Input: part model. Units: mm. Frame: model coordinates. A direction names the side the tool comes from. Round coordinates to 2 decimals unless told otherwise and drop trailing zeros. Loops run counter-clockwise (first coordinate to the right, second up) from the corner with the lowest first, then second, coordinate; pieces in that order, holes last. Notation, with made-up numbers: M -19,19.5 L 11,19.5 A11 ccw 11,26.5 Z; hole C 45,77.5 d5. An arc over 180 degrees is marked long. Put each result on its own line as item: value. Start each with the question number.
1) Line query: probe 1 along Y at (x, z) = (0, 18.75); probe 2 along Z at (x, y) = (-26, 22.5); probe 3 along X at (y, z) = (2.5, 0). Output: solid intervals per line, ascending.
2) Section D-D on x = 0. State how many separate pieces and enclosed holes the cut face has, plus the area to 3 significant figures.
3) Section C-C on x = 19. Output: boundary loops of the cut face in (y, z).
4) Section A-A on z = 0. Output: boundary loops of the cut face in (x, y), plus the area to 3 significant figures.
5) Pin query (flat end, axial travel): pin 1 (4 mm diameter, centred on y = 16.5, z = 15, fed in from -X); pin 2 (22 mm diameter, centred on x = 21, z = -1.5, fed in from +Y); pin 3 (16 mm diameter, centred on x = -21, z = 2, fed in from +Y). Return the tip coordinate at first contact, or that it passes through.
6) Draft query along Z for faces 1 (the face through (0, 15, 22.5)), 2 (the face through (22.057, 10.804, 15.789)), 3 (the face through (-8, 0, -15)). Return one class per face: +Z half, -Z half, draft (parallel to the pull), parting line (faces both ways), or undercut.
7) Reachability of faces 4 (the face through (19.2, 27.98, 20.04)), 5 (the face through (-21.775, 10.711, -15.696)) from +Z, -Z, +X, -X, +Y, -Y: full face, straight path, thin tool, end or side. Return the list, or none.
8) Section B-B on y = 22.22. Output: boundary loops of the cut face in (x, z).
Autodesk Fusion 360 part; units mm, degrees
sketch "Sketch1" plane through (0, 0, 0) normal (0, 1, 0) x (1, 0, 0)
  line L0 (32, -22.5) -> (-32, -22.5)
  line L1 (-32, -22.5) -> (-32, 22.5)
  line L2 (-32, 22.5) -> (32, 22.5)
  line L3 (32, 22.5) -> (32, -22.5)
  line L4 (32, -22.5) -> (-32, 22.5) construction
  line L5 (-32, -22.5) -> (32, 22.5) construction
  dimension "d1" = 64
  dimension "d6" = 45
extrude "Extrude1" add sketch "Sketch1" along normal blind 40
sketch "Sketch2" plane through (0, 0, 22.5) normal (0, 0, 1) x (-1, 0, 0)
  line L0 (32, 0) -> (-32, 0)
  line L1 (-32, 0) -> (-32, -40)
  line L2 (-32, -40) -> (32, -40)
  line L3 (32, -40) -> (32, 0)
  circle A0 centre (0, -29) radius 11
  line L4 (32, -16) -> (18.8835, -16)
  line L5 (18.8835, -16) -> (-32, -16)
  line L6 (6.7633, -37.6751) -> (32, -18)
  line L7 (-6.7633, -37.6751) -> (-32, -18)
  line L8 (0, 0) -> (0, -40) construction
  line L9 (32, -18) -> (-32, -18)
  dimension "d4" = 22
  dimension "d5" = 24
  dimension "d7" = 22
extrude "Extrude2" cut sketch "Sketch2" against normal blind 45 contours L2 L3 A0 L6 | L1 L2 A0 L7
sketch "Sketch3" plane through (-32, 0, 0) normal (-1, 0, 0) x (0, -1, 0)
  line L0 (-18, 22.5) -> (-18, -22.5)
  line L1 (-18, -22.5) -> (0, -22.5)
  line L2 (0, -22.5) -> (0, 22.5)
  line L3 (0, 22.5) -> (-18, 22.5)
  line L4 (0, 0) -> (-40.0524, 0)
  line L5 (-40, 22.5) -> (-40, -22.5)
  line L6 (-40, -22.5) -> (-37.6751, -22.5)
  line L7 (-37.6751, 22.5) -> (-40, 22.5)
  line L8 (-40, 17.5) -> (-9, 17.5)
  line L9 (-9, 17.5) -> (-9, -17.5)
  line L10 (-9, -17.5) -> (-40, -17.5)
  line L11 (-40, -17.5) -> (-40, 17.5)
  line L12 (-40, 17.5) -> (-9, -17.5) construction
  line L13 (-9, 17.5) -> (-40, -17.5) construction
  point P0 (-24.5, 0)
  dimension "d10" = 35
  dimension "d11" = 31
extrude "Extrude3" cut sketch "Sketch3" against normal blind 64 contours L0 L4 L8 L9 | L0 L4 L5 L8 L11 | L0 L4 L9 L10 | L0 L4 L5 L10 L11
sketch "Sketch4" plane through (0, 0, 22.5) normal (0, 0, 1) x (-1, 0, 0)
  line L0 (6.7633, -37.6751) -> (32, -18)
  line L1 (32, -18) -> (32, 0)
  line L2 (32, 0) -> (-32, 0)
  line L3 (-32, 0) -> (-32, -18)
  line L4 (-32, -18) -> (-6.7633, -37.6751)
  arc A0 (-6.7633, -37.6751) -> (6.7633, -37.6751) centre (0, -29) ccw
  circle A1 centre (0, -29) radius 11
  circle A2 centre (0, -29) radius 3.175
  line L5 (0, -40) -> (0, 0)
  point P0 (0, -34.92)
  point P1 (0, -22.22)
  dimension "d14" = 22
  dimension "d15" = 6.35
  dimension "d18" = 12.7
  dimension "d19" = 5.08
hole "Hole1" at (0, 22.22, 22.5) at (0, 34.92, 22.5) direction (0, 0, -1) diameter 6.5 depth 49 tip angle 180
sketch "Sketch5" plane through (0, 0, 0) normal (0, -1, 0) x (1, 0, 0)
  line L0 (-32, -22.5) -> (32, -22.5)
  line L1 (32, -22.5) -> (32, 22.5)
  line L2 (32, 22.5) -> (-32, 22.5)
  line L3 (-32, 22.5) -> (-32, -22.5)
  circle A0 centre (0, 0) radius 16.5
  dimension "d23" = 33
extrude "Extrude5" cut sketch "Sketch5" against normal blind 9 contours A0
fillet "Fillet1" radius 6 2 edges at (0, 9, -17.5) (0, 9, 17.5)
Geometry results:
1. probe 1: y = 0 to 18.97, 25.47 to 31.67, 38.17 to 40
1. probe 2: z = -22.5 to -17.5, 17.5 to 22.5
1. probe 3: x = -32 to -16.5, 16.5 to 32
2. separate pieces: 6
2. enclosed holes: 0
2. area: 290 mm²
3. outline: M 0,-22.5 L 28.14,-22.5 L 28.14,-17.5 L 15,-17.5 A6 cw 9,-11.5 L 9,11.5 A6 cw 15,17.5 L 28.14,17.5 L 28.14,22.5 L 0,22.5 Z
4. outline: M -32,0 L -16.5,0 L -16.5,9 L -32,9 Z; M 16.5,0 L 32,0 L 32,9 L 16.5,9 Z
4. area: 279 mm²
5. pin 1: passes through
5. pin 2: stops at y = 9.08
5. pin 3: stops at y = 9
6. face 1: +Z half
6. face 2: undercut
6. face 3: draft
7. face 4: +Z, -Z, +X, +Y
7. face 5: +X, -X, +Y
8. outline: M -26.59,-22.5 L -3.25,-22.5 L -3.25,-17.5 L -26.59,-17.5 Z; M -26.59,17.5 L -3.25,17.5 L -3.25,22.5 L -26.59,22.5 Z; M 3.25,-22.5 L 26.59,-22.5 L 26.59,-17.5 L 3.25,-17.5 Z; M 3.25,17.5 L 26.59,17.5 L 26.59,22.5 L 3.25,22.5 Z
